from build123d import *

# Parameters (mm, degrees)
SKETCH_W      = 120
SKETCH_H      = 90
PAD_DEPTH     = 4
SKETCH001_W   = 120
SKETCH001_H   = 90
SKETCH001_W_2 = 116
SKETCH001_H_2 = 86
PAD001_DEPTH  = 25
SKETCH002_W   = 3
SKETCH002_H   = 90
PAD002_DEPTH  = 20
SKETCH004_R   = 3
HOLE_DEPTH    = 25


with BuildPart() as part:
    # Sketch → Pad (new body)
    with BuildSketch(Plane.XZ):
        Rectangle(SKETCH_W, SKETCH_H)
    extrude(amount=PAD_DEPTH)

    # Sketch001 (on Face6 of Pad) → Pad001 (join)
    with BuildSketch(Plane.XZ.offset(4)):
        Rectangle(SKETCH001_W, SKETCH001_H)
        with Locations((0, -0.662812)):
            Rectangle(SKETCH001_W_2, SKETCH001_H_2, mode=Mode.SUBTRACT)
    extrude(amount=PAD001_DEPTH)

    # Sketch002 (on Face15 of Pad001) → Pad002 (join)
    with BuildSketch(Plane.XZ.offset(4)):
        with Locations((5, 0)):
            Rectangle(SKETCH002_W, SKETCH002_H)
    extrude(amount=PAD002_DEPTH)

    # Sketch004 (on Face14 of Pad002) → Hole (cut)
    with BuildSketch(Plane(origin=(0, 0, 42.337188), x_dir=(1, 0, 0), z_dir=(0, 0, -1))):
        with Locations((-47.758679, 14.860328)):
            Circle(SKETCH004_R)
    extrude(amount=-HOLE_DEPTH, mode=Mode.SUBTRACT)


solid = part.part
The listing builds one solid part. Answer for the finished solid, in the listing's coordinates (mm). A direction names the side the tool comes from. Coordinates: 2 decimals unless noted, no trailing zeros. Order: outer loops, then holes, each group sorted by start corner. A loop starts at its lowest first (then second) coordinate and runs counter-clockwise, first axis right, second up.
Q1. For a pull along X with two mould halves and no side action, classify faces 1 (the face through (-28, -4, 0)), 2 (the face through (-60, -14, -1)), 3 (the face through (-1, -14, 45)) as pulls with the +X half, pulls with the -X half, needs draft (parallel to the pull), parting line crosses it, or undercut.
Q2. A cutting plane is placed at B-B, the plane z = -35. Write down the section's boundary in (x, y), and give its area (3 significant figures).
Q3. A cutting plane is placed at C-C, the plane x = -20. Write down the section's boundary in (y, z), and give its area (3 significant figures).
Q4. Which of the six approach directions +Z, -Z, +X, -X, +Y, -Y give full straight-line access (tool end or side, diameter ignored) to faces 4 (the face through (-58, -16, -1)), 5 (the face through (-1, -14, -45)), 6 (the face through (-50.139, -13.035, 43.65))?
Q5. Given P1, Ø7, axis at x = -47.76, y = -14.86, coming from the +Z side; P2, Ø5, axis at x = -24.5, z = -31.5, coming from the -Y side; P3, Ø3.5, axis at x = 5, z = -11.5, coming from the -Y side, each flat-ended and moving along its own axis, determine where each tip first touches the part or whether it passes through.
Q6. A cutting plane is placed at A-A, the plane y = -6.25. Write down the section's boundary in (x, z), and give its area (3 significant figures).
Q7. Consider line 1 (X direction, y = -6, z = -14); line 2 (Z direction, x = -35, y = -11.75); line 3 (X direction, y = -24.25, z = 26.5). Determine where each line is inside the solid, lowest interval first.
Answers follow:
1. face 1: undercut
1. face 2: pulls with the -X half
1. face 3: needs draft
2. outline: (-60, -29) - (-58, -29) - (-58, -4) - (3.5, -4) - (3.5, -24) - (6.5, -24) - (6.5, -4) - (58, -4) - (58, -29) - (60, -29) - (60, 0) - (-60, 0) - close
2. area: 640 mm2
3. outline: (-29, -45) - (0, -45) - (0, 45) - (-29, 45) - (-29, 42.34) - (-4, 42.34) - (-4, -43.66) - (-29, -43.66) - close
3. area: 460 mm2
4. face 4: -Y
4. face 5: -Z, +X, -X, +Y, -Y
4. face 6: +Z
5. P1: stops at z = 45
5. P2: stops at y = -4
5. P3: stops at y = -24
6. outline: (-60, -45) - (60, -45) - (60, 45) - (-60, 45) - close; hole (-58, -43.66) - (3.5, -43.66) - (3.5, 42.34) - (-58, 42.34) - close; hole (6.5, -43.66) - (58, -43.66) - (58, 42.34) - (6.5, 42.34) - close
6. area: 1,080 mm2
7. line 1: x = -60 to -58, 3.5 to 6.5, 58 to 60
7. line 2: z = -45 to -43.66, 42.34 to 45
7. line 3: x = -60 to -58, 58 to 60
